The figure shows three views and two pictorial views of one solid part (mm, origin at its lowest corner). Answer the questions. Coordinates: 2 decimals unless noted, no trailing zeros. Order: outer loops, then holes, each group sorted by start corner. A loop starts at its lowest first (then second) coordinate and runs counter-clockwise, first axis right, second up. Notation, with made-up numbers: (61.5, -18.75) - (77.5, -18.75) arc R11 ccw to (77.5, -5.75) - close; hole circle Ø3 at (31.5, 8.5). An arc over 180 degrees is marked (long way). Use one line per item in the form item = value.
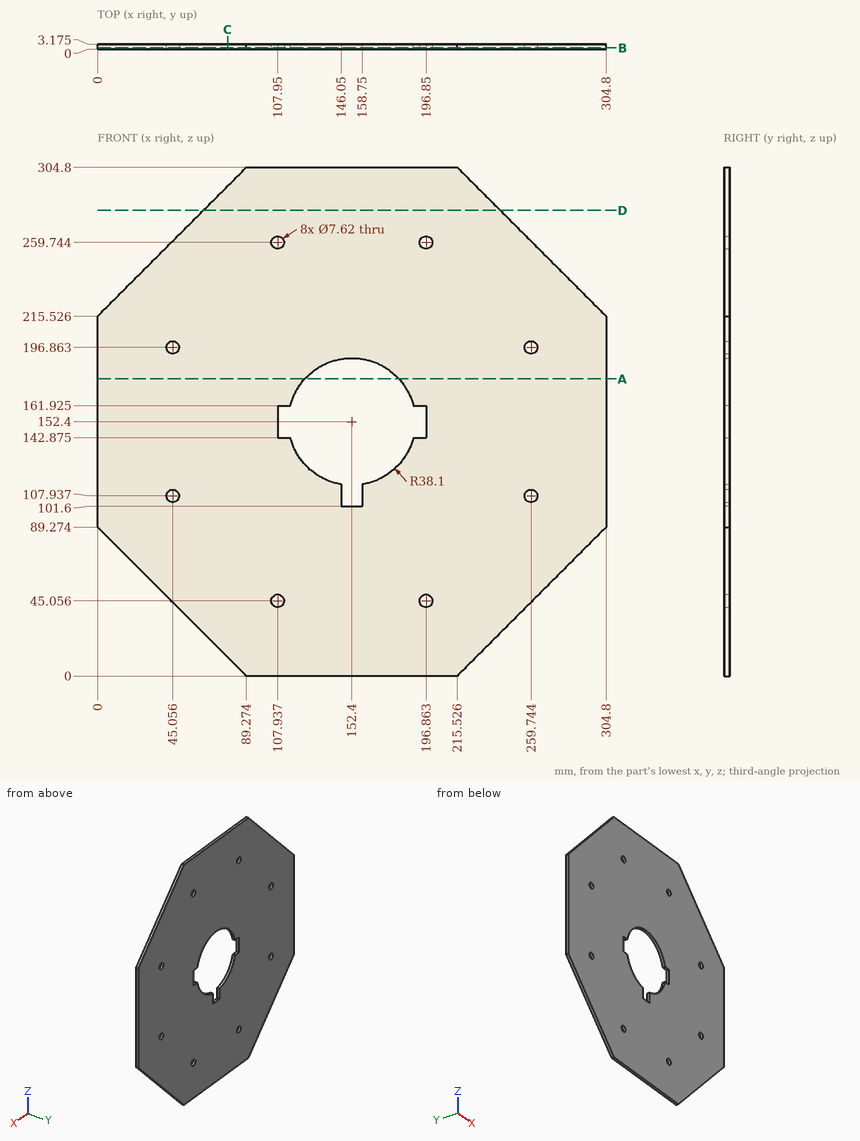
(1) Section A-A, the plane z = 178 is taken. Write down the section's boundary in (x, y) (1 decimal).
Answer list:
outline = (0, 0) - (124.2, 0) - (124.2, 3.2) - (0, 3.2) - close; (180.6, 0) - (304.8, 0) - (304.8, 3.2) - (180.6, 3.2) - close
(2) Section D-D, the plane z = 279 is taken. Write down the section's boundary in (x, y) (1 decimal).
Answer list:
outline = (63.5, 0) - (241.3, 0) - (241.3, 3.2) - (63.5, 3.2) - close
(3) Given pin 1 Ø1 at (x, y) = (229.5, 0.5) entering from +Z (1 decimal); pin 2 Ø1 at (x, y) = (71, 1) entering from +Z (1 decimal); pin 3 Ø1 at (x, y) = (237, 2) entering from +Z (1 decimal), each flat-ended and moving along its own axis, determine where each tip first touches the part or whether it passes through.
Answer list:
pin_1 = 291.3
pin_2 = 287
pin_3 = 283.8
(4) Section C-C, the plane x = 78 is taken. Write down the section's boundary in (y, z) (1 decimal).
Answer list:
outline = (0, 11.3) - (3.2, 11.3) - (3.2, 293.5) - (0, 293.5) - close
(5) Section B-B, the plane y = 0.9 is taken. State how many separate pieces and enclosed holes the cut face has, then the cut area to 3 significant figures.
Answer list:
separate_pieces = 1
enclosed_holes = 9
area = 71,600 mm2
(6) Straight lines are drawn through the part: L1, parallel to Z at x = 109, y = 2.9 (1 decimal); L2, parallel to X at y = 2.7, z = 149.5; L3, parallel to X at y = 2.8, z = 261.5 (1 decimal). For each, find the intervals that lie inside material, in ascending order.
Answer list:
L1 = 0 to 41.4, 48.7 to 142.9, 161.9 to 256.1, 263.4 to 304.8
L2 = 0 to 107.95, 196.85 to 304.8
L3 = 46 to 104.6, 111.3 to 193.5, 200.2 to 258.8
